```python
from build123d import *

# Parameters (mm, degrees)
F0_R          = 24.13
F0_R_2        = 20.447
F1_DEPTH      = 1308.1
F3_DEPTH      = 24.131
F3_DEPTH_BACK = 24.131
F5_DEPTH      = 24.131
F5_DEPTH_BACK = 24.131
F8_W          = 178.4191885963
F8_H          = 167.3920117319
F9_DEPTH      = 50.8
F9_DEPTH_BACK = 20.32


with BuildPart() as f1:
    # F0 (on Top) → F1 (new body)
    with BuildSketch(Plane.XY):
        Circle(F0_R)
        Circle(F0_R_2, mode=Mode.SUBTRACT)
    extrude(amount=F1_DEPTH)

    # F2 (on Right) → F3 (cut, two sides)
    with BuildSketch(Plane.YZ) as f3_sk:
        Polygon((24.13, 1288.3563127231), (24.13, 1308.1), (-24.13, 1308.1), align=None)
    extrude(amount=-F3_DEPTH, mode=Mode.SUBTRACT)
    extrude(f3_sk.sketch, amount=F3_DEPTH_BACK, mode=Mode.SUBTRACT)

    # F4 (on Front) → F5 (cut, two sides)
    with BuildSketch(Plane.XZ) as f5_sk:
        Polygon((-28.575, 0), (28.575, 0), (-28.575, 29.0972948719), align=None)
    extrude(amount=F5_DEPTH, mode=Mode.SUBTRACT)
    extrude(f5_sk.sketch, amount=-F5_DEPTH_BACK, mode=Mode.SUBTRACT)

    # F8 (on line) → F9 (cut, two sides)
    with BuildSketch(Plane(origin=(2.9412132624, -6.4824828952, 5.7768372862), x_dir=(-0.9471380058, -0.2395200516, 0.2134472836), z_dir=(-0.3208264297, 0.7071067812, -0.6301352252))) as f9_sk:
        with Locations((5.3417463787, 7.3568988591)):
            Rectangle(F8_W, F8_H)
    extrude(amount=F9_DEPTH, mode=Mode.SUBTRACT)
    extrude(f9_sk.sketch, amount=-F9_DEPTH_BACK, mode=Mode.SUBTRACT)


solid = f1.part
```
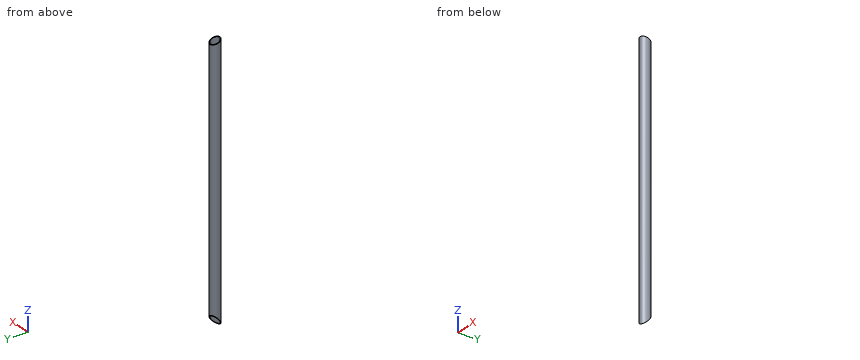
Can you work these out from the model? Positions are in its coordinate system, mm. Round coordinates to 2 decimals unless told otherwise and drop trailing zeros. Loops run counter-clockwise (first coordinate to the right, second up) from the corner with the lowest first, then second, coordinate; pieces in that order, holes last.
Item 1: Please list where these lines run through material, in increasing order: L1, parallel to Y at x = 0, z = 733; L2, parallel to Y at x = -9, z = 461.
Item 2: Suppose I cut it at C-C, the plane z = 407.5. Write out the boundary of the cut face in (x, y).
Item 3: Will these pins go through, and if not, where does the flat tip stop? pin 1 Ø1.5 at (y, z) = (5, 512) entering from +X; pin 2 Ø8 at (y, z) = (16, 592.5) entering from -X; pin 3 Ø10 at (x, z) = (19, 949) entering from +Y.
Item 4: Suppose I cut it at A-A, the plane y = 0. Write out the boundary of the cut face in (x, z).
Item 5: Suppose I cut it at B-B, the plane x = -8. Write out the boundary of the cut face in (y, z), then the cut area to 3 significant figures.
Reported:
1. L1: y = -24.13 to -20.45, 20.45 to 24.13
1. L2: y = -22.39 to -18.36, 18.36 to 22.39
2. outline: circle Ø48.26 at (0, 0); hole circle Ø40.89 at (0, 0)
3. pin 1: stops at x = 23.75
3. pin 2: stops at x = -20.93
3. pin 3: stops at y = 19.65
4. outline: (-24.13, 59.08) - (-20.45, 57.21) - (-20.45, 1298.23) - (-24.13, 1298.23) - close; (20.45, 36.39) - (24.13, 34.51) - (24.13, 1298.23) - (20.45, 1298.23) - close
5. outline: (-22.77, 25.32) - (-18.82, 29.75) - (-18.82, 1305.93) - (-22.77, 1307.54) - close; (18.82, 71.98) - (22.77, 76.41) - (22.77, 1288.91) - (18.82, 1290.53) - close
5. area: 9,850 mm2
